Verification items for the finished model (mm, model axes). A direction names the side the tool comes from. Coordinates: 2 decimals unless noted, no trailing zeros. Write each loop counter-clockwise with the first axis right and the second up, starting at its lowest first coordinate (ties: lowest second). Pieces come first, ordered by that corner, then holes. Notation, with made-up numbers: (47, 57.5) -> (93, 57.5) arc R28 ccw to (93, 96.5) -> close; hole circle Ø7 at (-14, 9). An arc over 180 degrees is marked (long way). Use a Markdown table: item, result. Add a question column.
from build123d import *

# Parameters (mm, degrees)
BOSS_EXTRUDE1_DEPTH = 3.175
BOSS_EXTRUDE2_DEPTH = 3.175
SKETCH2_W           = 12.7
SKETCH2_H           = 63.5
BOSS_EXTRUDE3_DEPTH = 2
CUT_EXTRUDE1_DEPTH  = 6.35
FILLET1_R           = 10


with BuildPart() as part:
    # Sketch1 → Boss-Extrude1 (new body)
    with BuildSketch(Plane.XY):
        with BuildLine():
            Line((12.586143856, 0), (52.341618497, 0))
            add(Edge.make_bspline(
                [(63.5, 15.783236994), (61.818196066, 5.163888879), (52.341618497, 0)],
                knots=[0, 0, 0, 1, 1, 1], degree=2))
            Line((63.5, 15.783236994), (63.5, 46.321965318))
            add(Edge.make_bspline(
                [(63.5, 46.321965318), (62.735953046, 56.152543933), (56.305780347, 63.5)],
                knots=[0, 0, 0, 1, 1, 1], degree=2))
            Line((56.305780347, 63.5), (6.82716763, 63.5))
            add(Edge.make_bspline(
                [(0, 46.321965318), (-0.299080934, 56.868733054), (6.82716763, 63.5)],
                knots=[0, 0, 0, 1, 1, 1], degree=2))
            Line((0, 46.321965318), (0, 15.783236994))
            add(Edge.make_bspline(
                [(0, 15.783236994), (0.304891955, 4.651584914), (12.586143856, 0)],
                knots=[0, 0, 0, 1, 1, 1], degree=2))
        make_face()
    extrude(amount=BOSS_EXTRUDE1_DEPTH)

    # Sketch3 → Boss-Extrude2 (add)
    with BuildSketch(Plane.XY.offset(3.175)):
        with BuildLine():
            Line((12.586143857, -1e-09), (52.341618497, 0))
            add(Edge.make_bspline(
                [(52.341618497, 0), (61.818196066, 5.163888879), (63.5, 15.783236995)],
                knots=[0, 0, 0, 1, 1, 1], degree=2))
            Line((63.5, 15.783236995), (63.5, 46.321965318))
            add(Edge.make_bspline(
                [(63.5, 46.321965318), (62.735953046, 56.152543933), (56.305780347, 63.5)],
                knots=[0, 0, 0, 1, 1, 1], degree=2))
            Line((56.305780347, 63.5), (6.82716763, 63.5))
            add(Edge.make_bspline(
                [(6.82716763, 63.5), (-0.299080929, 56.868733059), (0, 46.321965333)],
                knots=[0, 0, 0, 1, 1, 1], degree=2))
            Line((0, 46.321965333), (-2e-09, 15.783237047))
            add(Edge.make_bspline(
                [(-2e-09, 15.783237047), (0.304891926, 4.651584925), (12.586143857, -1e-09)],
                knots=[0, 0, 0, 1, 1, 1], degree=2))
        make_face()
    extrude(amount=BOSS_EXTRUDE2_DEPTH)

    # Sketch2 → Boss-Extrude3 (add)
    with BuildSketch(Plane(origin=(0, 0, 0), x_dir=(-1, 0, 0), z_dir=(0, 0, -1))):
        with Locations((-25.216473988, 31.75)):
            Rectangle(SKETCH2_W, SKETCH2_H)
        with Locations((-37.916473988, 31.75)):
            Rectangle(SKETCH2_W, SKETCH2_H)
    extrude(amount=BOSS_EXTRUDE3_DEPTH)

    # Sketch4 → Cut-Extrude1 (cut)
    with BuildSketch(Plane.XY.offset(6.35)):
        Polygon((47.703064377, 54.201225123), (50.44178546, 49.457621059), (55.919227626, 49.457621059), (58.657948709, 54.201225123), (55.919227626, 58.944829186), (50.44178546, 58.944829186), align=None)
        Polygon((36.950506543, 43.554276624), (39.690506543, 38.808457411), (45.170506543, 38.808457411), (47.910506543, 43.554276624), (45.170506543, 48.300095837), (39.690506543, 48.300095837), align=None)
        Polygon((47.703064377, 32.701225123), (50.44178546, 27.957621059), (55.919227626, 27.957621059), (58.657948709, 32.701225123), (55.919227626, 37.444829186), (50.44178546, 37.444829186), align=None)
        Polygon((36.950506543, 22.054276624), (39.690506543, 17.308457411), (45.170506543, 17.308457411), (47.910506543, 22.054276624), (45.170506543, 26.800095837), (39.690506543, 26.800095837), align=None)
        Polygon((47.703064377, 11.201225123), (50.44178546, 6.457621059), (55.919227626, 6.457621059), (58.657948709, 11.201225123), (55.919227626, 15.944829186), (50.44178546, 15.944829186), align=None)
        Polygon((26.203064377, 11.201225123), (28.94178546, 6.457621059), (34.419227626, 6.457621059), (37.157948709, 11.201225123), (34.419227626, 15.944829186), (28.94178546, 15.944829186), align=None)
        Polygon((26.203064377, 32.701225123), (28.94178546, 27.957621059), (34.419227626, 27.957621059), (37.157948709, 32.701225123), (34.419227626, 37.444829186), (28.94178546, 37.444829186), align=None)
        Polygon((26.203064377, 54.201225123), (28.94178546, 49.457621059), (34.419227626, 49.457621059), (37.157948709, 54.201225123), (34.419227626, 58.944829186), (28.94178546, 58.944829186), align=None)
        Polygon((15.450506543, 43.554276624), (18.190506543, 38.808457411), (23.670506543, 38.808457411), (26.410506543, 43.554276624), (23.670506543, 48.300095837), (18.190506543, 48.300095837), align=None)
        Polygon((4.703064377, 54.201225123), (7.44178546, 49.457621059), (12.919227626, 49.457621059), (15.657948709, 54.201225123), (12.919227626, 58.944829186), (7.44178546, 58.944829186), align=None)
        Polygon((4.703064377, 32.701225123), (7.44178546, 27.957621059), (12.919227626, 27.957621059), (15.657948709, 32.701225123), (12.919227626, 37.444829186), (7.44178546, 37.444829186), align=None)
        Polygon((15.450506543, 22.054276624), (18.190506543, 17.308457411), (23.670506543, 17.308457411), (26.410506543, 22.054276624), (23.670506543, 26.800095837), (18.190506543, 26.800095837), align=None)
        Polygon((4.703064377, 11.201225123), (7.44178546, 6.457621059), (12.919227626, 6.457621059), (15.657948709, 11.201225123), (12.919227626, 15.944829186), (7.44178546, 15.944829186), align=None)
    extrude(amount=-CUT_EXTRUDE1_DEPTH, mode=Mode.SUBTRACT)

    # Fillet1
    fillet1_edges = [part.edges().sort_by_distance(p)[0] for p in [
        (56.305780347, 63.5, 4.7625),
        (52.341618497, 0, 1.5875),
        (12.586143856, 0, 1.5875),
        (6.82716763, 63.5, 4.7625),
        (56.305780347, 63.5, 1.5875),
        (52.341618497, 0, 4.7625),
        (12.586143857, -1e-09, 4.7625),
        (6.82716763, 63.5, 1.5875),
    ]]
    fillet(fillet1_edges, radius=FILLET1_R)


solid = part.part
1) Gauge pin test, flat ends, axial feed: pin 1 (2 mm diameter, centred on x = 48.5, z = -0.5, fed in from -Y); pin 2 (3 mm diameter, centred on x = 33, y = 52.5, fed in from +Z); pin 3 (1.6 mm diameter, centred on y = 39, z = -1, fed in from -X); pin 4 (9.5 mm diameter, centred on x = 14, y = 23, fed in from -Z). Record the tip position at first contact, or that the pin passes through.
2) Cross-section at A-A on x = 41.5. Record the boundary of the cut face in (y, z) (3 decimals), then the cut area to 3 significant figures.
3) Release check for a two-part mould opening along X. For faces 1 (the face through (38.34, 45.96, 3.22)), 2 (the face through (18.866, 31, -1)) record: released by +X, released by -X, zero draft, split by the parting line, or undercut.
4) Set-up check for faces 3 (the face through (41, 22, 0)), 4 (the face through (53, 15.945, 3)): record each of +Z, -Z, +X, -X, +Y, -Y from which the full face is reachable in a straight line by a thin tool's end or side.
5) Cross-section at D-D on x = 25. Record the boundary of the cut face in (y, z) (3 decimals).
6) Cross-section at B-B on y = 25. Record the boundary of the cut face in (x, z) (3 decimals), then the cut area to 3 significant figures.
7) Thickness scan on L1, parallel to Y at x = 22, z = 0.5; L2, parallel to X at y = 53.5, z = 0.5; L3, parallel to Y at x = 16.5, z = 5.75. Record the ranges inside material, lowest first.
8) Cross-section at C-C on z = 1.5. Give the number of separate pieces and of enclosed holes in the cut face, then the cut area to 3 significant figures.
Returned:
| question | item | result |
|---|---|---|
| 1 | pin 1 | stops at y = 0 |
| 1 | pin 2 | stops at z = 0 |
| 1 | pin 3 | stops at x = 18.87 |
| 1 | pin 4 | stops at z = 0 |
| 2 | outline | (0, -2) -> (63.5, -2) -> (63.5, 6.35) -> (48.3, 6.35) -> (48.3, 0) -> (38.808, 0) -> (38.808, 6.35) -> (26.8, 6.35) -> (26.8, 0) -> (17.308, 0) -> (17.308, 6.35) -> (0, 6.35) -> close |
| 2 | area | 410 mm² |
| 3 | face 1 | undercut |
| 3 | face 2 | released by -X |
| 4 | face 3 | +Z |
| 4 | face 4 | +Z, -Z |
| 5 | outline | (0, -2) -> (63.5, -2) -> (63.5, 6.35) -> (45.997, 6.35) -> (45.997, 0) -> (41.111, 0) -> (41.111, 6.35) -> (24.497, 6.35) -> (24.497, 0) -> (19.611, 0) -> (19.611, 6.35) -> (0, 6.35) -> close |
| 6 | outline | (0, 0) -> (17.151, 0) -> (17.151, 6.35) -> (0, 6.35) -> close; (18.866, -2) -> (44.266, -2) -> (44.266, 0) -> (38.651, 0) -> (38.651, 6.35) -> (24.71, 6.35) -> (24.71, 0) -> (18.866, 0) -> close; (46.21, 0) -> (63.5, 0) -> (63.5, 6.35) -> (46.21, 6.35) -> close |
| 6 | area | 358 mm² |
| 7 | L1 | y = 0 to 17.31, 26.8 to 38.81, 48.3 to 63.5 |
| 7 | L2 | x = 0.77 to 5.11, 15.25 to 26.61, 36.75 to 48.11, 58.25 to 62.08 |
| 7 | L3 | y = 0 to 20.24, 23.87 to 41.74, 45.37 to 63.5 |
| 8 | separate pieces | 1 |
| 8 | enclosed holes | 13 |
| 8 | area | 2,820 mm² |
